```python
from build123d import *

# Parameters (mm, degrees)
SKETCH1_R           = 1.5
BOSS_EXTRUDE1_DEPTH = 5
SKETCH2_R           = 1.5
CUT_EXTRUDE1_DEPTH  = 5
CUT_EXTRUDE2_START  = -44
SKETCH2_2_R         = 1.5
CUT_EXTRUDE2_DEPTH  = 4


with BuildPart() as part:
    # Sketch1 → Boss-Extrude1 (new body)
    with BuildSketch(Plane(origin=(0, 0, 0), x_dir=(0, 0, -1), z_dir=(1, 0, 0))):
        with BuildLine():
            Line((-5.5, 20), (-5.5, -20))
            ThreePointArc((-5.5, -20), (-5.050348735, -22.178067412), (-3.774917218, -24))
            Line((-3.774917218, -24), (3.774917218, -24))
            ThreePointArc((3.774917218, -24), (5.050348735, -22.178067412), (5.5, -20))
            Line((5.5, -20), (5.5, 20))
            ThreePointArc((5.5, 20), (5.050348735, 22.178067412), (3.774917218, 24))
            Line((3.774917218, 24), (-3.774917218, 24))
            ThreePointArc((-3.774917218, 24), (-5.050348735, 22.178067412), (-5.5, 20))
        make_face()
        with Locations((0, 20)):
            Circle(SKETCH1_R, mode=Mode.SUBTRACT)
        with Locations((0, -15)):
            Circle(SKETCH1_R, mode=Mode.SUBTRACT)
    extrude(amount=BOSS_EXTRUDE1_DEPTH)

    # Sketch2 → Cut-Extrude1 (cut)
    with BuildSketch(Plane.XZ.offset(24)):
        with Locations(Location((2.5, 0, 0), (0, 0, 270))):
            Circle(SKETCH2_R)
    extrude(amount=-CUT_EXTRUDE1_DEPTH, mode=Mode.SUBTRACT)

    # Sketch2<2> → Cut-Extrude2 (cut)
    with BuildSketch(Plane.XZ.offset(24).offset(CUT_EXTRUDE2_START)):
        with Locations(Location((2.5, 0, 0), (0, 0, 270))):
            Circle(SKETCH2_2_R)
    extrude(amount=-CUT_EXTRUDE2_DEPTH, mode=Mode.SUBTRACT)


solid = part.part
```
Geometry: final body of the model. Coordinates: model frame, mm. A direction names the side the tool comes from. Round coordinates to 2 decimals unless told otherwise and drop trailing zeros. Order: outer loops, then holes, each group sorted by start corner. A loop starts at its lowest first (then second) coordinate and runs counter-clockwise, first axis right, second up. Notation, with made-up numbers: M 71,2.25 L 129,2.25 A24 cw 129,32.25 Z; hole C 77.5,-37 d7. An arc over 180 degrees is marked long. One line per item, written item: value.
(1) Cut plane D-D (z = -4.25). Return the cut outline in (x, y), and give its area (3 significant figures).
Result sheet:
outline: M 0,-23.49 L 5,-23.49 L 5,23.49 L 0,23.49 Z
area: 235 mm2
(2) Cut plane A-A (y = -15). Return the cut outline in (x, z).
Result sheet:
outline: M 0,-5.5 L 5,-5.5 L 5,-1.5 L 0,-1.5 Z; M 0,1.5 L 5,1.5 L 5,5.5 L 0,5.5 Z
(3) Cut plane C-C (x = 4.5). Return the cut outline in (y, z), and give its area (3 significant figures).
Result sheet:
outline: M -24,-3.77 A5.5 ccw -20,-5.5 L 20,-5.5 A5.5 ccw 24,-3.77 L 24,3.77 A5.5 ccw 20,5.5 L -20,5.5 A5.5 ccw -24,3.77 Z; hole C -15,0 d3; hole C 20,0 d3
area: 505 mm2
(4) Line query: probe 1 along Y at (x, z) = (2, 0); probe 2 along X at (y, z) = (-20.35, 0); probe 3 along Z at (x, y) = (4.45, 20.5). Output: solid intervals per line, ascending. Write a range as [from, to].
Result sheet:
probe 1: [-19, -16.5], [-13.5, 18.5]
probe 2: [0, 1], [4, 5]
probe 3: [-5.48, -1.41], [1.41, 5.48]
(5) Pull-direction query (Z, two-part tool) for faces 4 (the cylindrical face through (2.465, 22.149, -5.063)), 5 (the cylindrical face through (2.465, 18.536, 0.325)), 6 (the flat face through (2, 0, 5.5)); classes: pulls with the +Z half, pulls with the -Z half, needs draft (parallel to the pull), parting line crosses it, or undercut.
Result sheet:
face 4: pulls with the -Z half
face 5: undercut
face 6: pulls with the +Z half
(6) Pin query (flat end, axial travel): P1, Ø3, axis at y = -15.5, z = -0.5, coming from the -X side; P2, Ø2.5, axis at x = 2.5, z = 0, coming from the +Y side; P3, Ø2.5, axis at x = 2.5, z = 0, coming from the -Y side. Return the tip coordinate at first contact, or that it passes through.
Result sheet:
P1: x = 0
P2: y = 19.17
P3: y = -19
(7) Cut plane B-B (x = 2.5). Return the cut outline in (y, z), and give its area (3 significant figures).
Result sheet:
outline: M -24,-3.77 A5.5 ccw -20,-5.5 L 20,-5.5 A5.5 ccw 24,-3.77 L 24,-1.5 L 20,-1.5 A1.5 cw 20,1.5 L 24,1.5 L 24,3.77 A5.5 ccw 20,5.5 L -20,5.5 A5.5 ccw -24,3.77 L -24,1.5 L -19,1.5 L -19,-1.5 L -24,-1.5 Z; hole C -15,0 d3
area: 482 mm2
(8) Reachability of faces 1 (the cylindrical face through (2.57, 22.42, 1.5)), 2 (the flat face through (3, -19, 0)), 3 (the flat face through (0.8, 24, -0.1)) from +Z, -Z, +X, -X, +Y, -Y: full face, straight path, thin tool, end or side. Return the list, or none.
Result sheet:
face 1: +Y
face 2: -Y
face 3: +Z, -Z, +X, -X, +Y
